For this review, take the finished solid that the model builds, in its own axes (mm). A direction names the side the tool comes from. Round coordinates to 2 decimals unless told otherwise and drop trailing zeros. Order: outer loops, then holes, each group sorted by start corner. A loop starts at its lowest first (then second) coordinate and runs counter-clockwise, first axis right, second up. Notation, with made-up numbers: (19, 13.25) - (38, 13.25) arc R22 ccw to (38, 42.25) - close; hole circle Ø6 at (0.5, -12). An arc over 180 degrees is marked (long way). One line per item, written item: value.
```python
from build123d import *

# Parameters (mm, degrees)
ESQUISSE2_R        = 1
BOSS_EXTRU_1_DEPTH = 4.9
CHANFREIN1_SIZE    = 0.1


with BuildPart() as part:
    # Esquisse1 → R_volution1 (revolve)
    with BuildSketch(Plane.XY, mode=Mode.PRIVATE) as r_volution1_sk:
        with BuildLine():
            Line((-1.75, -39.787533784), (-1.75, 39.787533784))
            ThreePointArc((-1.75, 39.787533784), (-2.749195521, 43.022997284), (0, 45))
            Line((0, 45), (0, -45))
            ThreePointArc((0, -45), (-2.749195521, -43.022997284), (-1.75, -39.787533784))
        make_face()
    revolve(r_volution1_sk.sketch.rotate(Axis((0, 45, 0), (0, -1, 0)), 270), axis=Axis((0, 45, 0), (0, -1, 0)))

    # Esquisse2 → Boss.-Extru.1 (add, symmetric)
    with BuildSketch(Plane(origin=(0, 0, 0), x_dir=(0, 0, -1), z_dir=(1, 0, 0))):
        with Locations((0, 42.1)):
            Circle(ESQUISSE2_R)
    boss_extru_1 = extrude(amount=BOSS_EXTRU_1_DEPTH, both=True)

    # Sym_trie3: Boss.-Extru.1 across plane
    add(boss_extru_1.mirror(Plane.ZX))

    # Chanfrein1
    chanfrein1_edges = [part.edges().sort_by_distance(p)[0] for p in [
        (-4.9, 42.1, 1),
        (4.9, 42.1, 1),
        (4.9, -42.1, 1),
        (-4.9, -42.1, 1),
    ]]
    chamfer(chanfrein1_edges, length=CHANFREIN1_SIZE)


solid = part.part
```
Item 1: Take a section at B-B (z = 0). Write out the cut boundary in (x, y), plus the area to 3 significant figures.
Returned:
outline: (-4.9, -43) - (-4.8, -43.1) - (-2.72, -43.1) arc R2.9 ccw to (2.72, -43.1) - (4.8, -43.1) - (4.9, -43) - (4.9, -41.2) - (4.8, -41.1) - (2.72, -41.1) arc R2.9 ccw to (1.75, -39.79) - (1.75, 39.79) arc R2.9 ccw to (2.72, 41.1) - (4.8, 41.1) - (4.9, 41.2) - (4.9, 43) - (4.8, 43.1) - (2.72, 43.1) arc R2.9 ccw to (-2.72, 43.1) - (-4.8, 43.1) - (-4.9, 43) - (-4.9, 41.2) - (-4.8, 41.1) - (-2.72, 41.1) arc R2.9 ccw to (-1.75, 39.79) - (-1.75, -39.79) arc R2.9 ccw to (-2.72, -41.1) - (-4.8, -41.1) - (-4.9, -41.2) - close
area: 345 mm^2
Item 2: Take a section at C-C (x = 3.5). Write out the cut boundary in (y, z).
Returned:
outline: circle Ø2 at (-42.1, 0); circle Ø2 at (42.1, 0)
Item 3: Take a section at A-A (y = 42.1). Write out the cut boundary in (x, z).
Returned:
outline: (-4.9, -0.9) - (-4.8, -1) - (-2.72, -1) arc R2.9 ccw to (2.72, -1) - (4.8, -1) - (4.9, -0.9) - (4.9, 0.9) - (4.8, 1) - (2.72, 1) arc R2.9 ccw to (-2.72, 1) - (-4.8, 1) - (-4.9, 0.9) - close
Item 4: The part is to be moulded in two halves that separate along Y. For faces 1 (the flat face through (-4.9, 42, 0)), 2 (the cylindrical face through (1.71, 0.56, -0.38)), say which applies: +Y half, -Y half, draft (parallel to the pull), parting line (faces both ways), or undercut.
Returned:
face 1: draft
face 2: undercut
Item 5: Wall thickness on line 1 (Z direction, x = 1.5, y = 38.5); line 2 (Y direction, x = -4, z = -0.6); line 3 (Y direction, x = 4, z = -0.9): over which ranges is each line inside the solid? List them lowest first.
Returned:
line 1: -0.9 to 0.9
line 2: -42.9 to -41.3, 41.3 to 42.9
line 3: -42.54 to -41.66, 41.66 to 42.54
Item 6: Machinability: for faces 3 (the cylindrical face through (3.78, -43.09, 0.13)), 4 (the cylindrical face through (-3.75, 43.09, 0.13)), 5 (the flat face through (4.9, -42, 0)), which of the approach directions +Z, -Z, +X, -X, +Y, -Y give a long, thin tool a straight path to every point of the face, cutting with its end or side? Answer none if there is none.
Returned:
face 3: +X
face 4: -X
face 5: +Z, -Z, +X, +Y, -Y
Item 7: Take a section at D-D (x = 0). Write out the cut boundary in (y, z), plus the area to 3 significant figures.
Returned:
outline: (-39.79, -1.75) - (39.79, -1.75) arc R2.9 ccw (long way) to (39.79, 1.75) - (-39.79, 1.75) arc R2.9 ccw (long way) to start
area: 329 mm^2
Item 8: For P1, Ø1.5, axis at y = 25, z = -0.5, coming from the +X side; P2, Ø1.5, axis at y = 6.5, z = -1.5, coming from the +X side; P3, Ø2, axis at y = -25, z = 2, coming from the +X side, all flat-tipped, find the tip position at first contact; note any pin that passes through.
Returned:
P1: x = 1.75
P2: x = 1.58
P3: x = 1.44
